```python
from build123d import *

# Parameters (mm, degrees)
F0_W     = 965.2
F0_H     = 711.2
F1_DEPTH = 12.7
F2_W     = 965.2
F2_H     = 711.2
F2_W_2   = 939.8
F2_H_2   = 685.8
F3_DEPTH = 406.4


with BuildPart() as f1:
    # F0 (on Top) → F1 (new body)
    with BuildSketch(Plane.XY):
        with Locations((482.6, -355.6)):
            Rectangle(F0_W, F0_H)
    extrude(amount=-F1_DEPTH)

    # F2 (on face) → F3 (join)
    with BuildSketch(Plane(origin=(0, 0, -12.7), x_dir=(1, 0, 0), z_dir=(0, 0, -1))):
        with Locations((482.6, 355.6)):
            Rectangle(F2_W, F2_H)
        with Locations((482.6, 355.6)):
            Rectangle(F2_W_2, F2_H_2, mode=Mode.SUBTRACT)
    extrude(amount=F3_DEPTH)


solid = f1.part
```
Check sheet for the modelled part. Datum: model origin and axes. Units: mm. A direction names the side the tool comes from. Coordinates: 2 decimals unless noted, no trailing zeros. Loops run counter-clockwise (first coordinate to the right, second up) from the corner with the lowest first, then second, coordinate; pieces in that order, holes last.
1) Access from +Z, -Z, +X, -X, +Y, -Y to the whole of each face (thin tool, end or side, straight path). Record for faces 1 (the face through (952.5, -351, -213)), 2 (the face through (480, -700, -419.1)).
2) Gauge pin test, flat end, axial feed: pin 1 (6 mm diameter, centred on x = 113, y = -81.5, fed in from -Z). Record the tip position at first contact, or that the pin passes through.
3) Release check for a two-part mould opening along X. For faces 3 (the face through (476, -711.2, -207)), 4 (the face through (965.2, -351, -207)), 5 (the face through (476, -698.5, -213)) record: released by +X, released by -X, zero draft, split by the parting line, or undercut.
4) Sectioned sample at C-C (x = 675). Record the boundary of the cut face in (y, z).
5) Sectioned sample at B-B (y = -59.5). Record the boundary of the cut face in (x, z), and give its area (3 significant figures).
6) Material ranges on probe 1 along Y at (x, z) = (634.5, -248); probe 2 along X at (y, z) = (-555.5, -305.5); probe 3 along Z at (x, y) = (391.5, -281), recorded low to high.
7) Sectioned sample at A-A (z = -141.5). Record the boundary of the cut face in (x, y).
Check sheet entries:
1. face 1: -Z
1. face 2: -Z, +X, -X, +Y, -Y
2. pin 1: stops at z = -12.7
3. face 3: zero draft
3. face 4: released by +X
3. face 5: undercut
4. outline: (-711.2, -419.1) - (-698.5, -419.1) - (-698.5, -12.7) - (-12.7, -12.7) - (-12.7, -419.1) - (0, -419.1) - (0, 0) - (-711.2, 0) - close
5. outline: (0, -419.1) - (12.7, -419.1) - (12.7, -12.7) - (952.5, -12.7) - (952.5, -419.1) - (965.2, -419.1) - (965.2, 0) - (0, 0) - close
5. area: 22,600 mm2
6. probe 1: y = -711.2 to -698.5, -12.7 to 0
6. probe 2: x = 0 to 12.7, 952.5 to 965.2
6. probe 3: z = -12.7 to 0
7. outline: (0, -711.2) - (965.2, -711.2) - (965.2, 0) - (0, 0) - close; hole (12.7, -698.5) - (952.5, -698.5) - (952.5, -12.7) - (12.7, -12.7) - close
